Input: part model. Units: mm. Frame: model coordinates. A direction names the side the tool comes from. Round coordinates to 2 decimals unless told otherwise and drop trailing zeros. Order: outer loops, then holes, each group sorted by start corner. A loop starts at its lowest first (then second) coordinate and runs counter-clockwise, first axis right, second up. Notation, with made-up numbers: (36, 20.5) - (86, 20.5) arc R21 ccw to (86, 32.5) - close; hole circle Ø4 at (-17.75, 12). An arc over 180 degrees is marked (long way). One line per item, written item: value. Start each with the question number.
Solid Edge part; units mm, degrees
sketch "Sketch1" plane through (0, 0, 0) normal (1, 0, 0) x (0, 1, 0)
  line L0 (-70.6829, -147.8929) -> (-40.6829, -147.8929)
  line L1 (-40.6829, -147.8929) -> (-40.6829, 12.1071)
  line L2 (-40.6829, 12.1071) -> (-70.6829, 12.1071)
  line L3 (-70.6829, 12.1071) -> (-70.6829, -147.8929)
  line L4 (-70.6829, 12.1071) -> (-40.6829, 12.1071)
  line L5 (-54.1753, 28.1984) -> (-40.6829, 12.1071)
  line L6 (-57.1901, 28.1988) -> (-54.1753, 28.1984)
  line L7 (-70.6829, 12.1071) -> (-57.1901, 28.1988)
  dimension "D1" = 70.6829
  dimension "D2" = 54.1753
  dimension "D3" = 70.6829
  dimension "D4" = 40.6829
  dimension "D5" = 40.6829
  dimension "D6" = 0
extrude "Protrusion1" add sketch "Sketch1" against normal blind 3
sketch "Sketch2" plane through (0, -21.8205, 20.1807) normal (1, 0, 0) x (0, 1, 0)
  circle A0 centre (-33.8621, -1.9821) radius 5
  dimension "D1" = 33.8621
  dimension "D2" = 33.8621
extrude "ExtrudedProtrusion_2" add sketch "Sketch2" along normal blind 11
mirror "Mirror1" about plane through (5, -21.8205, 20.1506) normal (1, 0, 0) of "Protrusion1"
sketch "Sketch3" plane through (11.5, -70.6829, -27.8929) normal (0, -1, 0) x (0, 0, -1)
  arc A0 (120, -1.5) -> (120, -11.5) centre (168.482, -6.5) ccw
  line L0 (115, -1.5) -> (120, -1.5)
  arc A1 (115, -1.5) -> (115, -11.5) centre (164.7494, -6.5) ccw
  line L1 (120, -11.5) -> (115, -11.5)
  dimension "D1" = 115
extrude "ExtrudedProtrusion_4" add sketch "Sketch3" against normal blind 30
Item 1: Reachability of faces 1 (the face through (4.93, -59.65, 21.24)), 2 (the face through (5.07, -55.893, -142.642)), 3 (the face through (-1, -56, -147.893)) from +Z, -Z, +X, -X, +Y, -Y: full face, straight path, thin tool, end or side. Return the list, or none.
Item 2: Line query: L1, parallel to X at y = -68.5, z = -100.5; L2, parallel to Z at x = 5.25, y = -48; L3, parallel to Z at x = 7, y = -57. Output: solid intervals per line, ascending.
Item 3: Section query D-D on x = -1.5. Return loops of the section in (y, z), and give its area (3 significant figures).
Item 4: Section query C-C on y = -64. Return loops of the section in (x, z).
Item 5: First-contact query: pin 1 Ø4 at (x, y) = (5.5, -58) entering from +Z. Flat tip, straight axial feed; report the tip coordinate or a pass-through.
Item 6: Section query B-B on x = 8.5. Return loops of the section in (y, z), and give its area (3 significant figures).
Item 7: Pull-direction query (X, two-part tool) for faces 4 (the face through (13, -56, -59)), 5 (the face through (10, -56, -56)), 6 (the face through (11.5, -47.3, 20)); classes: released by +X, released by -X, zero draft, split by the parting line, or undercut.
Item 8: Section query A-A on z = -87. Return loops of the section in (x, y), and give its area (3 significant figures).
Geometry results:
1. face 1: none
1. face 2: +Y, -Y
1. face 3: -Z, +X, -X, +Y, -Y
2. L1: x = -3 to 0, 10 to 13
2. L2: z = -147.64 to -142.64
2. L3: z = -147.68 to -142.68, 13.38 to 23.02
3. outline: (-70.68, -147.89) - (-40.68, -147.89) - (-40.68, 12.11) - (-54.18, 28.2) - (-57.19, 28.2) - (-70.68, 12.11) - close
3. area: 5,070 mm^2
4. outline: (-3, -147.89) - (0, -147.89) arc R48.74 cw to (10, -147.89) - (13, -147.89) - (13, 20.08) - (10, 20.08) - (10, -142.89) arc R50 ccw to (0, -142.89) - (0, 20.08) - (-3, 20.08) - close
5. pin 1: stops at z = 23.19
6. outline: (-70.68, -147.76) - (-40.68, -147.76) - (-40.68, -142.76) - (-70.68, -142.76) - close; circle Ø10 at (-55.68, 18.2)
6. area: 228 mm^2
7. face 4: released by +X
7. face 5: undercut
7. face 6: zero draft
8. outline: (-3, -70.68) - (0, -70.68) - (0, -40.68) - (-3, -40.68) - close; (10, -70.68) - (13, -70.68) - (13, -40.68) - (10, -40.68) - close
8. area: 180 mm^2
